The model under review builds one solid part; all positions refer to its coordinate system, in mm. Face numbers are marked on the shaded views. A direction names the side the tool comes from. Give positions to 0.01 mm unless a question says otherwise; leave off trailing zeros. Write each loop counter-clockwise with the first axis right and the second up, starting at its lowest first coordinate (ties: lowest second). Pieces come first, ordered by that corner, then holes. Notation, with made-up numbers: (47, 86.25) - (88, 86.25) arc R19 ccw to (88, 106.25) - close; hole circle Ø11 at (81, -21). An arc over 180 degrees is marked (long way). Write item = value, one per line.
```python
from build123d import *

# Parameters (mm, degrees)
F1_DEPTH     = 101.6
F2_R         = 5.08
F3_R         = 5.08
F4_T1_DEPTH  = 28.8312589727
F4_T4_ANGLE  = 250.1936024552
F4_T6_ANGLE  = 35.0968012276
F4_T8_ANGLE  = 35.0968012276
F4_T10_ANGLE = 35.0968012276
F4_T12_ANGLE = 35.0968012276
F4_T14_ANGLE = 250.1936024552


# Not quite as in the source:
# - a fillet or chamfer that OpenCascade refuses, or shapes differently, is made with other operations: its cross-section is extruded or revolved along the edge and cut away or added


with BuildPart() as f1:
    # F0 (on Front) → F1 (new body)
    with BuildSketch(Plane.XZ):
        with BuildLine():
            Line((16.1115902063, 17.78), (-16.1115902063, 17.78))
            ThreePointArc((-16.1115902063, 17.78), (-53.34, 0), (-16.1115902063, -17.78))
            Line((-16.1115902063, -17.78), (16.1115902063, -17.78))
            ThreePointArc((16.1115902063, -17.78), (53.34, 0), (16.1115902063, 17.78))
        make_face()
        with BuildLine():
            ThreePointArc((-12.7, 0), (0, 12.7), (12.7, 0))
            ThreePointArc((12.7, 0), (0, -12.7), (-12.7, 0))
        make_face(mode=Mode.SUBTRACT)
    extrude(amount=F1_DEPTH)

    # F2
    f2_edges = [f1.edges().sort_by_distance(p)[0] for p in [
        (-16.11159, -50.8, 17.78),
        (16.11159, -50.8, 17.78),
    ]]
    fillet(f2_edges, radius=F2_R)

    # F3
    f3_edges = [f1.edges().sort_by_distance(p)[0] for p in [
        (-16.11159, -50.8, -17.78),
        (16.11159, -50.8, -17.78),
    ]]
    fillet(f3_edges, radius=F3_R)

    # F4: chamfer of 5.08 on 9 edges, made by hand

    # F4_s2 → F4_t1 (cut)
    with BuildSketch(Plane.YZ.offset(-14.4156294863)):
        Polygon((-96.52, -17.78), (-101.6, -12.7), (-101.6, -17.78), align=None)
        Polygon((-96.52, 17.78), (-101.6, 12.7), (-101.6, 17.78), align=None)
    extrude(amount=F4_T1_DEPTH, mode=Mode.SUBTRACT)

    # F4_s3 → F4_t4 (revolve, cut)
    with BuildSketch(Plane(origin=(20.4039669421, 0, -14.3384464089), x_dir=(0, 1, 0), z_dir=(-0.8181818182, 0, 0.5749595746))):
        Polygon((-96.52, 5.3352321669), (-101.6, 0.2552321669), (-101.6, 5.3352321669), align=None)
    revolve(axis=Axis((30.48, -101.6, 0), (0, -1, 0)), revolution_arc=F4_T4_ANGLE, mode=Mode.SUBTRACT)

    # F4_s5 → F4_t6 (revolve, cut)
    with BuildSketch(Plane(origin=(20.4039669421, 0, -14.3384464089), x_dir=(0, 1, 0), z_dir=(0.8181818182, 0, -0.5749595746))):
        Polygon((-96.52, -5.3352321669), (-101.6, -0.2552321669), (-101.6, -5.3352321669), align=None)
    revolve(axis=Axis((14.4156294863, -101.6, -22.86), (0, -1, 0)), revolution_arc=F4_T6_ANGLE, mode=Mode.SUBTRACT)

    # F4_s7 → F4_t8 (revolve, cut)
    with BuildSketch(Plane.YZ.offset(14.4156294863)):
        Polygon((-96.52, 17.78), (-101.6, 12.7), (-101.6, 17.78), align=None)
    revolve(axis=Axis((14.4156294863, -101.6, 22.86), (0, -1, 0)), revolution_arc=F4_T8_ANGLE, mode=Mode.SUBTRACT)

    # F4_s9 → F4_t10 (revolve, cut)
    with BuildSketch(Plane(origin=(-20.4039669421, 0, -14.3384464089), x_dir=(0, 1, 0), z_dir=(-0.8181818182, 0, -0.5749595746))):
        Polygon((-96.52, 5.3352321669), (-101.6, 0.2552321669), (-101.6, 5.3352321669), align=None)
    revolve(axis=Axis((-14.4156294863, -101.6, -22.86), (0, 1, 0)), revolution_arc=F4_T10_ANGLE, mode=Mode.SUBTRACT)

    # F4_s11 → F4_t12 (revolve, cut)
    with BuildSketch(Plane.YZ.offset(-14.4156294863)):
        Polygon((-96.52, 17.78), (-101.6, 12.7), (-101.6, 17.78), align=None)
    revolve(axis=Axis((-14.4156294863, -101.6, 22.86), (0, 1, 0)), revolution_arc=F4_T12_ANGLE, mode=Mode.SUBTRACT)

    # F4_s13 → F4_t14 (revolve, cut)
    with BuildSketch(Plane(origin=(-20.4039669421, 0, 14.3384464089), x_dir=(0, 1, 0), z_dir=(0.8181818182, 0, -0.5749595746))):
        Polygon((-96.52, 5.3352321669), (-101.6, 0.2552321669), (-101.6, 5.3352321669), align=None)
    revolve(axis=Axis((-30.48, -101.6, 0), (0, -1, 0)), revolution_arc=F4_T14_ANGLE, mode=Mode.SUBTRACT)

    # F4_s15 → F4_t16 (revolve, cut)
    with BuildSketch(Plane.XY):
        Polygon((12.7, -96.52), (17.78, -101.6), (12.7, -101.6), align=None)
    revolve(axis=Axis((0, -101.6, 0), (0, -1, 0)), mode=Mode.SUBTRACT)


solid = f1.part
```
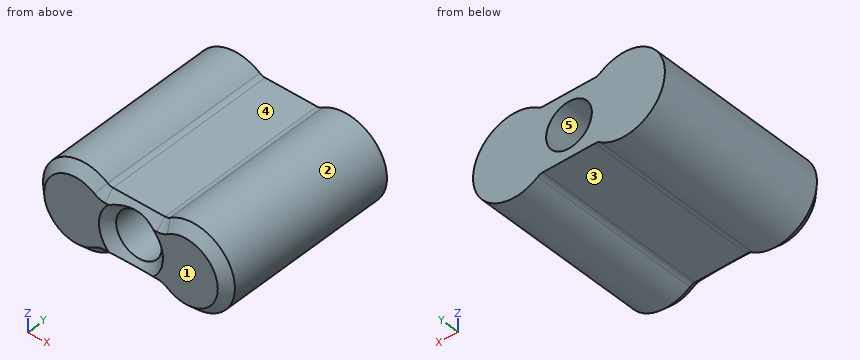
1. For line 1 (Z direction, x = 0, y = -45); line 2 (X direction, y = -40.5, z = 0); line 3 (X direction, y = -95.5, z = 3.5), list the stretches that pass through material, from the lowest coordinate up. Write a range as from..to.
Findings below:
line_1 = -17.78..-12.7, 12.7..17.78
line_2 = -53.34..-12.7, 12.7..53.34
line_3 = -53.07..-12.21, 12.21..53.07
2. Take a section at C-C on x = 0. Give the boundary of the cut face in (y, z).
Findings below:
outline = (-99.06, -15.24) - (-96.52, -17.78) - (0, -17.78) - (0, -12.7) - (-96.52, -12.7) - close; (-99.06, 15.24) - (-96.52, 12.7) - (0, 12.7) - (0, 17.78) - (-96.52, 17.78) - close
3. Insertion check: P1, Ø8.5, axis at x = -5.5, y = -36.5, coming from the -Z side; P2, Ø3, axis at x = 40, y = -14.5, coming from the -Z side; P3, Ø5, axis at x = -6.5, z = -17, coming from the -Y side. Each pin has a flat end and moves straight along its axis. Give the tip position at first contact, or say it passes through.
Findings below:
P1 = -17.78
P2 = -21.41
P3 = -99.79
4. Take a section at B-B on y = -21. Give the boundary of the cut face in (x, z), and give its area (3 significant figures).
Findings below:
outline = (-17.34, -18.7) arc R5.08 cw to (-14.42, -17.78) - (14.42, -17.78) arc R5.08 cw to (17.34, -18.7) arc R22.86 ccw (long way) to (17.34, 18.7) arc R5.08 cw to (14.42, 17.78) - (-14.42, 17.78) arc R5.08 cw to (-17.34, 18.7) arc R22.86 ccw (long way) to start; hole circle Ø25.4 at (0, 0)
area = 3,500 mm²
5. Machinability: for the marked faces 3, 4 and 5, which of the approach directions +Z, -Z, +X, -X, +Y, -Y give a long, thin tool a straight path to every point of the face, cutting with its end or side? Answer none if there is none.
Findings below:
face_3 = -Z, +Y, -Y
face_4 = +Z, +Y, -Y
face_5 = +Y, -Y
6. Draft analysis for pull direction X (two halves, no side actions). For the marked faces 1 and 2, state which applies: +X half, -X half, draft (parallel to the pull), parting line (faces both ways), or undercut.
Findings below:
face_1 = draft
face_2 = undercut
7. Take a section at A-A on z = 0. Give the boundary of the cut face in (x, y), and give its area (3 significant figures).
Findings below:
outline = (-53.34, -96.52) - (-48.26, -101.6) - (-17.78, -101.6) - (-12.7, -96.52) - (-12.7, 0) - (-53.34, 0) - close; (12.7, -96.52) - (17.78, -101.6) - (48.26, -101.6) - (53.34, -96.52) - (53.34, 0) - (12.7, 0) - close
area = 8,210 mm²
